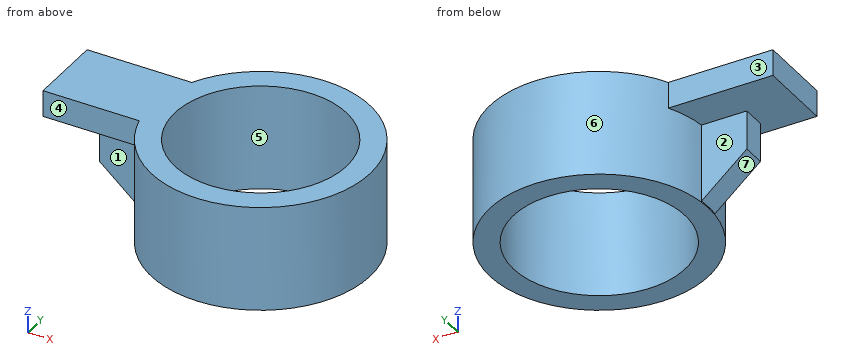
from build123d import *

# Parameters (mm, degrees)
F0_R     = 26.313439
F1_DEPTH = 25.4
F3_R     = 20.660218
F4_DEPTH = 25.401
F5_DEPTH = 6.35
F6_W     = 10.94192
F6_H     = 5.624315
F7_DEPTH = 18.796
F9_DEPTH = 29.034779


with BuildPart() as f1:
    # F0 (on Top) → F1 (new body)
    with BuildSketch(Plane.XY):
        with Locations((21.762719, -2.72034)):
            Circle(F0_R)
    extrude(amount=F1_DEPTH)

    # F3 (on face) → F4 (cut, through all)
    with BuildSketch(Plane(origin=(0, 0, 0), x_dir=(1, 0, 0), z_dir=(0, 0, -1))):
        with Locations((21.762719, 2.72034)):
            Circle(F3_R)
    extrude(amount=-F4_DEPTH, mode=Mode.SUBTRACT)

    # F2 (on face) → F5 (join)
    with BuildSketch(Plane.XY.offset(25.4)):
        with BuildLine():
            ThreePointArc((-3.75248, -9.15242), (-4.389986, 0.183635), (-1.719926, 9.15242))
            Line((-1.719926, 9.15242), (-26.911331, 9.15242))
            Line((-26.911331, 9.15242), (-26.911331, -9.15242))
            Line((-26.911331, -9.15242), (-3.75248, -9.15242))
        make_face()
    extrude(amount=-F5_DEPTH)

    # F6 (on face) → F7 (join)
    with BuildSketch(Plane(origin=(0, 0, 19.05), x_dir=(1, 0, 0), z_dir=(0, 0, -1))):
        with Locations((-9.860946, 2.812158)):
            Rectangle(F6_W, F6_H)
    extrude(amount=F7_DEPTH)

    # F8 (on face) → F9 (cut, through all)
    with BuildSketch(Plane(origin=(0, 0, 0), x_dir=(-1, 0, 0), z_dir=(0, 1, 0))):
        Polygon((15.331906, 0.254), (15.331906, 9.652), (4.409725, 0.254), align=None)
    extrude(amount=-F9_DEPTH, mode=Mode.SUBTRACT)


solid = f1.part
Check sheet for the modelled part. Datum: model origin and axes. Units: mm. Face numbers are marked on the shaded views. A direction names the side the tool comes from. Give positions to 0.01 mm unless a question says otherwise; leave off trailing zeros. Loops run counter-clockwise (first coordinate to the right, second up) from the corner with the lowest first, then second, coordinate; pieces in that order, holes last. Notation, with made-up numbers: M -3.5,-26.75 L 52.5,-26.75 A16 cw 52.5,-20.75 Z; hole C 49.5,24 d6. An arc over 180 degrees is marked long. Return JSON: item names as keys, results as strings. Group by question number.
1. Cross-section at C-C on z = 3.25. Record the boundary of the cut face in (x, y).
2. Cross-section at A-A on x = 29.5. Record the boundary of the cut face in (y, z).
3. Cross-section at B-B on y = -19. Record the boundary of the cut face in (x, z).
4. Go/stop test with flat-tipped pins: pin 1 (4.5 mm diameter, centred on y = -1.5, z = 15, fed in from -X); pin 2 (9 mm diameter, centred on x = -10, y = -4, fed in from -Z); pin 3 (5 mm diameter, centred on x = -10, z = 22, fed in from -Y). Record where each tip stops, or that it passes through.
5. Thickness scan on L1, parallel to Z at x = -14.5, y = 6.5; L2, parallel to X at y = 12, z = 5.5; L3, parallel to X at y = 5.5, z = 12.75. Record the ranges inside material, lowest first.
6. Mould release check, pull along X, two halves, no side actions. Record for the marked faces 5, 6 and 7: released by +X, released by -X, zero draft, split by the parting line, or undercut.
7. Cross-section at D-D on x = -5.5. Record the boundary of the cut face in (y, z).
8. Tool access check on the marked faces 1, 2, 3 and 4. Record the directions out of +Z, -Z, +X, -X, +Y, -Y that give a thin tool (end or side, any length) a straight path to the whole face; none if there is none.
Return value:
{
 "1": {"outline": "M -7.89,-5.62 L -4.39,-5.62 A26.31 ccw long -4.41,0 L -7.89,0 Z; hole C 21.76,-2.72 d41.32"},
 "2": {"outline": "M -27.87,0 L -21.88,0 L -21.88,25.4 L -27.87,25.4 Z; M 16.44,0 L 22.43,0 L 22.43,25.4 L 16.44,25.4 Z"},
 "3": {"outline": "M 1.09,0 L 9.04,0 L 9.04,25.4 L 1.09,25.4 Z; M 34.48,0 L 42.44,0 L 42.44,25.4 L 34.48,25.4 Z"},
 "4": {"pin 1": "x = -15.33", "pin 2": "z = 1.19", "pin 3": "y = -9.15"},
 "5": {"L1": "19.05 to 25.4", "L2": "-0.05 to 7.27, 36.26 to 43.57", "L3": "-3.23 to 2.81, 40.72 to 46.76"},
 "6": {"face 5": "undercut", "face 6": "split by the parting line", "face 7": "released by -X"},
 "7": {"outline": "M -9.15,19.05 L -5.62,19.05 L -5.62,1.19 L 0,1.19 L 0,19.05 L 9.15,19.05 L 9.15,25.4 L -9.15,25.4 Z"},
 "8": {"face 1": "-Z, -X, -Y", "face 2": "-Z, -X, +Y", "face 3": "+Z, -Z, -X, +Y", "face 4": "+Z, -Z, -X, -Y"}
}
